Here's how the part is built. I have some questions about the finished solid (model axes, mm). A direction names the side the tool comes from. Round coordinates to 2 decimals unless told otherwise and drop trailing zeros. Write each loop counter-clockwise with the first axis right and the second up, starting at its lowest first coordinate (ties: lowest second). Pieces come first, ordered by that corner, then holes. Notation, with made-up numbers: (3.5, 31) - (12.5, 31) arc R31 cw to (12.5, 62) - close; hole circle Ø5 at (-29, 3). An arc over 180 degrees is marked (long way). One line per item, written item: value. Start each with the question number.
Item 1: Imagine slicing it at B-B, the plane x = -7.5. Please give me the cut outline in (y, z), then the cut area to 3 significant figures.
Item 2: Thinking about a two-plate mould opening in Z: for faces 1 (the face through (78.295, -0.362, -74.102)), 2 (the face through (79.01, -12.86, 74.67)), 3 (the face through (5, -11, -35.56)), which applies, released by +Z, released by -Z, zero draft, split by the parting line, or undercut?
Item 3: Imagine slicing it at C-C, the plane y = -11.25. Please give me the cut outline in (x, z), then the cut area to 3 significant figures.
Item 4: If I drill on line 1 (X direction, y = -13.75, z = 36) (3 decimals); line 2 (Z direction, x = 10.5, y = -18.25); line 3 (X direction, y = -3.5, z = -35), over which ranges is the centre line in solid material (lowest first)?
Item 5: For faces 4 (the face through (-69.83, -25.06, -74.02)), 5 (the face through (3.94, -22.9, 38.14)), 6 (the face through (4, -11, 35.56)), which set-ups out of +Z, -Z, +X, -X, +Y, -Y let a thin tool reach every point of the face, with its end or its side?
Item 6: Imagine slicing it at A-A, the plane z = -8. Please give me the cut outline in (x, y).
Item 7: Imagine slicing it at D-D, the plane x = 43. Count the separate pieces of the cut face and the enclosed holes in it, then the cut area to 3 significant figures.
```python
from build123d import *

# Parameters (mm, degrees)
F1_DEPTH = 25.4
F2_SIZE  = 5.08
F3_R     = 5.08
F4_SIZE  = 1.27


with BuildPart() as f1:
    # F0 (on Front) → F1 (new body)
    with BuildSketch(Plane.XZ):
        with BuildLine():
            Line((-31.3017520181, 76.2), (-71.9417520181, 76.2))
            Line((-71.9417520181, 76.2), (-71.9417520181, 35.56))
            Line((-71.9417520181, 35.56), (-44.0017520181, 35.56))
            ThreePointArc((-44.0017520181, 35.56), (-40.2820081392, 44.5402561211), (-31.3017520181, 48.26))
            Line((-31.3017520181, 48.26), (-31.3017520181, 76.2))
        make_face()
        with BuildLine():
            Line((80.4582479819, 76.2), (-31.3017520181, 76.2))
            Line((-31.3017520181, 76.2), (-31.3017520181, 48.26))
            ThreePointArc((-31.3017520181, 48.26), (-22.3214958971, 44.5402561211), (-18.6017520181, 35.56))
            Line((-18.6017520181, 35.56), (27.1226329476, 35.56))
            ThreePointArc((27.1226329476, 35.56), (30.8423768265, 44.5402561211), (39.8226329476, 48.26))
            ThreePointArc((39.8226329476, 48.26), (48.8028890686, 44.5402561211), (52.5226329476, 35.56))
            Line((52.5226329476, 35.56), (80.4582479819, 35.56))
            Line((80.4582479819, 35.56), (80.4582479819, 76.2))
        make_face()
        with BuildLine():
            Line((-44.0017520181, 35.56), (-71.9417520181, 35.56))
            Line((-71.9417520181, 35.56), (-71.9417520181, -35.56))
            Line((-71.9417520181, -35.56), (-44.0017520181, -35.56))
            ThreePointArc((-44.0017520181, -35.56), (-40.2820081392, -26.5797438789), (-31.3017520181, -22.86))
            Line((-31.3017520181, -22.86), (-31.3017520181, 22.86))
            ThreePointArc((-31.3017520181, 22.86), (-40.2820081392, 26.5797438789), (-44.0017520181, 35.56))
        make_face()
        with BuildLine():
            Line((-44.0017520181, -35.56), (-71.9417520181, -35.56))
            Line((-71.9417520181, -35.56), (-71.9417520181, -76.2))
            Line((-71.9417520181, -76.2), (-31.3017520181, -76.2))
            Line((-31.3017520181, -76.2), (-31.3017520181, -48.26))
            ThreePointArc((-31.3017520181, -48.26), (-40.2820081392, -44.5402561211), (-44.0017520181, -35.56))
        make_face()
        with BuildLine():
            Line((80.4582479819, -35.56), (80.4582479819, 35.56))
            Line((80.4582479819, 35.56), (52.5226329476, 35.56))
            ThreePointArc((52.5226329476, 35.56), (48.8028890686, 26.5797438789), (39.8226329476, 22.86))
            Line((39.8226329476, 22.86), (39.8226329476, -22.86))
            ThreePointArc((39.8226329476, -22.86), (48.8028890686, -26.5797438789), (52.5226329476, -35.56))
            Line((52.5226329476, -35.56), (80.4582479819, -35.56))
        make_face()
        with BuildLine():
            Line((80.4582479819, -76.2), (80.4582479819, -35.56))
            Line((80.4582479819, -35.56), (52.5226329476, -35.56))
            ThreePointArc((52.5226329476, -35.56), (48.8028890686, -44.5402561211), (39.8226329476, -48.26))
            Line((39.8226329476, -48.26), (39.8226329476, -76.2))
            Line((39.8226329476, -76.2), (80.4582479819, -76.2))
        make_face()
        with BuildLine():
            Line((-31.3017520181, -48.26), (-31.3017520181, -76.2))
            Line((-31.3017520181, -76.2), (39.8226329476, -76.2))
            Line((39.8226329476, -76.2), (39.8226329476, -48.26))
            ThreePointArc((39.8226329476, -48.26), (30.8423768265, -44.5402561211), (27.1226329476, -35.56))
            Line((27.1226329476, -35.56), (-18.6017520181, -35.56))
            ThreePointArc((-18.6017520181, -35.56), (-22.3214958971, -44.5402561211), (-31.3017520181, -48.26))
        make_face()
    extrude(amount=F1_DEPTH)

    # F2
    f2_edges = [f1.edges().sort_by_distance(p)[0] for p in [
        (39.822633, -25.4, 0),
        (4.26044, -25.4, 35.56),
        (4.26044, -25.4, -35.56),
        (48.802889, -25.4, 44.540256),
        (48.802889, -25.4, -44.540256),
        (-40.282008, -25.4, -44.540256),
        (-31.301752, -25.4, 0),
        (-40.282008, -25.4, 44.540256),
    ]]
    chamfer(f2_edges, length=F2_SIZE)

    # F3
    f3_edges = [f1.edges().sort_by_distance(p)[0] for p in [
        (80.458248, -12.7, 76.2),
        (80.458248, -12.7, -76.2),
        (-71.941752, -12.7, -76.2),
        (-71.941752, -12.7, 76.2),
    ]]
    fillet(f3_edges, radius=F3_R)

    # F4
    f4_edges = [f1.edges().sort_by_distance(p)[0] for p in [
        (4.258248, -25.4, 76.2),
        (-71.941752, 0, 0),
        (4.26044, 0, 35.56),
        (-40.282008, 0, 44.540256),
        (-31.301752, 0, 0),
        (39.822633, 0, 0),
        (48.802889, 0, 44.540256),
        (4.26044, 0, -35.56),
        (-40.282008, 0, -44.540256),
        (48.802889, 0, -44.540256),
    ]]
    chamfer(f4_edges, length=F4_SIZE)


solid = f1.part
```
Values follow:
1. outline: (-25.4, -74.93) - (-24.13, -76.2) - (-1.27, -76.2) - (0, -74.93) - (0, -36.83) - (-1.27, -35.56) - (-20.32, -35.56) - (-25.4, -40.64) - close; (-25.4, 40.64) - (-20.32, 35.56) - (-1.27, 35.56) - (0, 36.83) - (0, 74.93) - (-1.27, 76.2) - (-24.13, 76.2) - (-25.4, 74.93) - close
1. area: 2,030 mm^2
2. face 1: released by -Z
2. face 2: released by +Z
2. face 3: undercut
3. outline: (-71.94, -71.12) arc R5.08 ccw to (-66.86, -76.2) - (75.38, -76.2) arc R5.08 ccw to (80.46, -71.12) - (80.46, 71.12) arc R5.08 ccw to (75.38, 76.2) - (-66.86, 76.2) arc R5.08 ccw to (-71.94, 71.12) - close; hole (-31.3, -22.86) arc R12.7 ccw (long way) to (-18.6, -35.56) - (27.12, -35.56) arc R12.7 ccw (long way) to (39.82, -22.86) - (39.82, 22.86) arc R12.7 ccw (long way) to (27.12, 35.56) - (-18.6, 35.56) arc R12.7 ccw (long way) to (-31.3, 22.86) - close
3. area: 16,600 mm^2
4. line 1: x = -71.942 to -43.994, -18.609 to 27.13, 52.515 to 80.458
4. line 2: z = -76.2 to -35.56, 35.56 to 76.2
4. line 3: x = -71.94 to -43.99, 52.51 to 80.46
5. face 4: -Z, -X, -Y
5. face 5: -Y
5. face 6: +Y, -Y
6. outline: (-71.94, -24.13) - (-70.67, -25.4) - (-36.38, -25.4) - (-31.3, -20.32) - (-31.3, -1.27) - (-32.57, 0) - (-70.67, 0) - (-71.94, -1.27) - close; (39.82, -20.32) - (44.9, -25.4) - (79.19, -25.4) - (80.46, -24.13) - (80.46, -1.27) - (79.19, 0) - (41.09, 0) - (39.82, -1.27) - close
7. separate pieces: 3
7. enclosed holes: 0
7. area: 2,490 mm^2
